Can you work these out from the model? Positions are in its coordinate system, mm. Face numbers are marked on the shaded views. Coordinates: 2 decimals unless noted, no trailing zeros. Order: outer loops, then holes, each group sorted by start corner. A loop starts at its lowest first (then second) coordinate and runs counter-clockwise, first axis right, second up. Notation, with made-up numbers: (-24.75, 39) - (17.25, 39) arc R20 ccw to (17.25, 65) - close; hole circle Ø3 at (7, -13.5). An arc over 180 degrees is marked (long way). Use a Markdown table: item, result. Add a question column.
(1) We'd pull the mould along Z, two halves only. Please class the marked faces 1, 2 and 3: pulls with the +Z half, pulls with the -Z half, needs draft (parallel to the pull), parting line crosses it, or undercut.
(2) If I drill on L1, parallel to Y at x = -12, z = 5; L2, parallel to X at y = 3, z = -3.5; L3, parallel to X at y = 2, z = 14.05, over which ranges is the centre line in solid material (lowest first)? Write a range as [from, to].
(3) For pin 1 Ø1.2 at (y, z) = (1, -12.5) entering from -X; pin 2 Ø1.5 at (y, z) = (1.5, 0) entering from +X; pin 3 Ø1.5 at (x, y) = (-11.5, 1) entering from +Z; pin 4 Ø10 at (x, z) = (-1, -7.5) entering from -Y, each with a flat end and sliding along its axis, tell me the tip position at first contact or that it passes through.
(4) I want a section at B-B (y = 0.75). List the corners of the cut face in (x, z) for me.
```python
from build123d import *

# Parameters (mm, degrees)
EXTRUDE_1_DEPTH          = 4
CUT_EXTRUDE_1_DEPTH      = 31.6757233
CUT_EXTRUDE_1_DEPTH_BACK = 31.6757233
SKETCH_2_R               = 0.5
CUT_EXTRUDE_2_REACH      = 32.237
SKETCH_3_R               = 0.5
FILLET_1_R               = 2
FILLET_2_R               = 1


# Some blends are built 0.0001 mm under size
with BuildPart() as part:
    # Эскиз1 → Бобышка-Вытянуть1 (new body)
    with BuildSketch(Plane(origin=(0, 0, 0), x_dir=(1, 0, 0), z_dir=(0, 1, 0))):
        Polygon((-10, 15), (10, 15), (10, 12), (5, 12), (5, -12), (10, -12), (10, -15), (-10, -15), (-10, -11.5), (-14, -11.5), (-14, 11.5), (-10, 11.5), align=None)
    extrude(amount=EXTRUDE_1_DEPTH)

    # Эскиз2 → Вырез-Вытянуть1 (cut, two sides: drawn at the far end of the back side and taken through both)
    with BuildSketch(Plane.XY.offset(-12).offset(-CUT_EXTRUDE_1_DEPTH_BACK)):
        with Locations((8, 2)):
            Circle(SKETCH_2_R)
    extrude(amount=CUT_EXTRUDE_1_DEPTH + CUT_EXTRUDE_1_DEPTH_BACK, mode=Mode.SUBTRACT)

    # Эскиз3 → Вырез-Вытянуть2 (cut, up to next)
    with BuildSketch(Plane.XY.offset(11.5), mode=Mode.PRIVATE) as cut_extrude_2_sk1:
        with Locations((-12, 2)):
            Circle(SKETCH_3_R)
    cut_extrude_2_tool1 = extrude(cut_extrude_2_sk1.sketch, amount=-CUT_EXTRUDE_2_REACH, mode=Mode.PRIVATE) & part.part
    add(cut_extrude_2_tool1.solids().sort_by_distance((-12, 2, 11.5))[0], mode=Mode.SUBTRACT)

    # Скругление1
    fillet_1_edges = [part.edges().sort_by_distance(p)[0] for p in [
        (10, 0, -13.5),
        (10, 4, -13.5),
        (10, 0, 13.5),
        (10, 4, 13.5),
        (-14, 0, 0),
        (-14, 4, 0),
        (-10, 2, -15),
        (-10, 2, 15),
    ]]
    fillet(fillet_1_edges, radius=FILLET_1_R - 0.0001)  # a hair under: the kernel refuses the full size

    # Скругление2
    # the kernel refuses this fillet: 1 mm, written as the material it takes off along each edge
    with BuildSketch(Plane(origin=(5, 4, -12), x_dir=(-1, 0, 0), z_dir=(0, 0, 1))) as fillet_2_piece_1:
        with BuildLine():
            CenterArc((FILLET_2_R, FILLET_2_R), FILLET_2_R, 180, 90)
            Line((0, FILLET_2_R), (0, 0))
            Line((0, 0), (FILLET_2_R, 0))
        make_face()
    extrude(amount=24, mode=Mode.SUBTRACT)
    with BuildSketch(Plane(origin=(10.5001, 4, -12), x_dir=(0, 0, -1), z_dir=(-1, 0, 0)), Plane(origin=(5, 4, 12), x_dir=(0, 0, 1), z_dir=(1, 0, 0))) as fillet_2_piece_2:
        with BuildLine():
            CenterArc((FILLET_2_R, FILLET_2_R), FILLET_2_R, 180, 90)
            Line((0, FILLET_2_R), (0, 0))
            Line((0, 0), (FILLET_2_R, 0))
        make_face()
    extrude(amount=5.5001, mode=Mode.SUBTRACT)
    with BuildSketch(Plane(origin=(-14.5001, 4, -11.5), x_dir=(0, 0, 1), z_dir=(1, 0, 0)), Plane(origin=(-10, 4, 11.5), x_dir=(0, 0, -1), z_dir=(-1, 0, 0))) as fillet_2_piece_3:
        with BuildLine():
            CenterArc((FILLET_2_R, FILLET_2_R), FILLET_2_R, 180, 90)
            Line((0, FILLET_2_R), (0, 0))
            Line((0, 0), (FILLET_2_R, 0))
        make_face()
    extrude(amount=4.5001, mode=Mode.SUBTRACT)
    with BuildSketch(Plane(origin=(-10, 4, 13.0001), x_dir=(1, 0, 0), z_dir=(0, 0, -1)), Plane(origin=(-10, 4, -11.5), x_dir=(1, 0, 0), z_dir=(0, 0, -1))) as fillet_2_piece_4:
        with BuildLine():
            CenterArc((FILLET_2_R, FILLET_2_R), FILLET_2_R, 180, 90)
            Line((0, FILLET_2_R), (0, 0))
            Line((0, 0), (FILLET_2_R, 0))
        make_face()
    extrude(amount=1.5001, mode=Mode.SUBTRACT)
    with BuildSketch(Plane(origin=(-8.0001, 4, -15), x_dir=(0, -1, 0), z_dir=(1, 0, 0))) as fillet_2_piece_5:
        with BuildLine():
            CenterArc((FILLET_2_R, -FILLET_2_R), FILLET_2_R, 90, 90)
            Line((0, -FILLET_2_R), (0, 0))
            Line((0, 0), (FILLET_2_R, 0))
        make_face()
    extrude(amount=18.5002, mode=Mode.SUBTRACT)
    with BuildSketch(Plane(origin=(10.5001, 4, 15), x_dir=(0, 0, -1), z_dir=(-1, 0, 0))) as fillet_2_piece_6:
        with BuildLine():
            CenterArc((FILLET_2_R, FILLET_2_R), FILLET_2_R, 180, 90)
            Line((0, FILLET_2_R), (0, 0))
            Line((0, 0), (FILLET_2_R, 0))
        make_face()
    extrude(amount=18.5002, mode=Mode.SUBTRACT)
    with BuildSketch(Plane(origin=(-8.0001, 4, 13.0001), x_dir=(0, 0, 1), z_dir=(1, 0, 0))) as fillet_2_piece_7:
        with BuildLine():
            CenterArc((1.9999 - FILLET_2_R, FILLET_2_R), FILLET_2_R, 270, 90)
            Line((1.9999, FILLET_2_R), (1.9999, 0))
            Line((1.9999, 0), (1.9999 - FILLET_2_R, 0))
        make_face()
    revolve(axis=Axis((-8.0001, 4, 13.0001), (0, -1, 0)), revolution_arc=90, mode=Mode.SUBTRACT)
    with BuildSketch(Plane(origin=(-8.0001, 4, -13.0001), x_dir=(0, 0, -1), z_dir=(1, 0, 0))) as fillet_2_piece_8:
        with BuildLine():
            CenterArc((1.9999 - FILLET_2_R, -FILLET_2_R), FILLET_2_R, 0, 90)
            Line((1.9999 - FILLET_2_R, 0), (1.9999, 0))
            Line((1.9999, 0), (1.9999, -FILLET_2_R))
        make_face()
    revolve(axis=Axis((-8.0001, 4, -13.0001), (0, 1, 0)), revolution_arc=90, mode=Mode.SUBTRACT)
    with BuildSketch(Plane(origin=(10.5001, 4, -12), x_dir=(0, 0, -1), z_dir=(-1, 0, 0))) as fillet_2_piece_9a_section:
        with BuildLine():
            CenterArc((FILLET_2_R, FILLET_2_R), FILLET_2_R, 180, 90)
            Line((0, FILLET_2_R), (0, 0))
            Line((0, 0), (FILLET_2_R, 0))
        make_face()
    fillet_2_piece_9a = extrude(amount=8.0001, mode=Mode.PRIVATE)
    fillet_2_piece_9a = split(fillet_2_piece_9a, bisect_by=Plane(origin=(5, 3.773604886, -12.226395114), z_dir=(-1, 0, 0)), keep=Keep.TOP, mode=Mode.PRIVATE)
    with BuildSketch(Plane(origin=(5, 4, -14.5), x_dir=(-1, 0, 0), z_dir=(0, 0, 1))) as fillet_2_piece_9b_section:
        with BuildLine():
            CenterArc((FILLET_2_R, FILLET_2_R), FILLET_2_R, 180, 90)
            Line((0, FILLET_2_R), (0, 0))
            Line((0, 0), (FILLET_2_R, 0))
        make_face()
    fillet_2_piece_9b = extrude(amount=26.5, mode=Mode.PRIVATE)
    fillet_2_piece_9b = split(fillet_2_piece_9b, bisect_by=Plane(origin=(4.773604886, 3.773604886, -12), z_dir=(0, 0, -1)), keep=Keep.TOP, mode=Mode.PRIVATE)
    fillet_2_piece_9 = fillet_2_piece_9a & fillet_2_piece_9b
    add(fillet_2_piece_9, mode=Mode.SUBTRACT)
    with BuildSketch(Plane(origin=(5, 4, -12), x_dir=(-1, 0, 0), z_dir=(0, 0, 1))) as fillet_2_piece_10a_section:
        with BuildLine():
            CenterArc((FILLET_2_R, FILLET_2_R), FILLET_2_R, 180, 90)
            Line((0, FILLET_2_R), (0, 0))
            Line((0, 0), (FILLET_2_R, 0))
        make_face()
    fillet_2_piece_10a = extrude(amount=26.5, mode=Mode.PRIVATE)
    fillet_2_piece_10a = split(fillet_2_piece_10a, bisect_by=Plane(origin=(4.773604886, 3.773604886, 12), z_dir=(0, 0, 1)), keep=Keep.TOP, mode=Mode.PRIVATE)
    with BuildSketch(Plane(origin=(2.5, 4, 12), x_dir=(0, 0, 1), z_dir=(1, 0, 0))) as fillet_2_piece_10b_section:
        with BuildLine():
            CenterArc((FILLET_2_R, FILLET_2_R), FILLET_2_R, 180, 90)
            Line((0, FILLET_2_R), (0, 0))
            Line((0, 0), (FILLET_2_R, 0))
        make_face()
    fillet_2_piece_10b = extrude(amount=8.0001, mode=Mode.PRIVATE)
    fillet_2_piece_10b = split(fillet_2_piece_10b, bisect_by=Plane(origin=(5, 3.773604886, 12.226395114), z_dir=(-1, 0, 0)), keep=Keep.TOP, mode=Mode.PRIVATE)
    fillet_2_piece_10 = fillet_2_piece_10a & fillet_2_piece_10b
    add(fillet_2_piece_10, mode=Mode.SUBTRACT)
    with BuildSketch(Plane(origin=(-10, 4, -9), x_dir=(1, 0, 0), z_dir=(0, 0, -1))) as fillet_2_piece_11a_section:
        with BuildLine():
            CenterArc((FILLET_2_R, FILLET_2_R), FILLET_2_R, 180, 90)
            Line((0, FILLET_2_R), (0, 0))
            Line((0, 0), (FILLET_2_R, 0))
        make_face()
    fillet_2_piece_11a = extrude(amount=4.0001, mode=Mode.PRIVATE)
    fillet_2_piece_11a = split(fillet_2_piece_11a, bisect_by=Plane(origin=(-9.773604886, 3.773604886, -11.5), z_dir=(0, 0, 1)), keep=Keep.TOP, mode=Mode.PRIVATE)
    with BuildSketch(Plane(origin=(-14.5001, 4, -11.5), x_dir=(0, 0, 1), z_dir=(1, 0, 0))) as fillet_2_piece_11b_section:
        with BuildLine():
            CenterArc((FILLET_2_R, FILLET_2_R), FILLET_2_R, 180, 90)
            Line((0, FILLET_2_R), (0, 0))
            Line((0, 0), (FILLET_2_R, 0))
        make_face()
    fillet_2_piece_11b = extrude(amount=7.0001, mode=Mode.PRIVATE)
    fillet_2_piece_11b = split(fillet_2_piece_11b, bisect_by=Plane(origin=(-10, 3.773604886, -11.273604886), z_dir=(1, 0, 0)), keep=Keep.TOP, mode=Mode.PRIVATE)
    fillet_2_piece_11 = fillet_2_piece_11a & fillet_2_piece_11b
    add(fillet_2_piece_11, mode=Mode.SUBTRACT)
    with BuildSketch(Plane(origin=(-7.5, 4, 11.5), x_dir=(0, 0, -1), z_dir=(-1, 0, 0))) as fillet_2_piece_12a_section:
        with BuildLine():
            CenterArc((FILLET_2_R, FILLET_2_R), FILLET_2_R, 180, 90)
            Line((0, FILLET_2_R), (0, 0))
            Line((0, 0), (FILLET_2_R, 0))
        make_face()
    fillet_2_piece_12a = extrude(amount=7.0001, mode=Mode.PRIVATE)
    fillet_2_piece_12a = split(fillet_2_piece_12a, bisect_by=Plane(origin=(-10, 3.773604886, 11.273604886), z_dir=(1, 0, 0)), keep=Keep.TOP, mode=Mode.PRIVATE)
    with BuildSketch(Plane(origin=(-10, 4, 13.0001), x_dir=(1, 0, 0), z_dir=(0, 0, -1))) as fillet_2_piece_12b_section:
        with BuildLine():
            CenterArc((FILLET_2_R, FILLET_2_R), FILLET_2_R, 180, 90)
            Line((0, FILLET_2_R), (0, 0))
            Line((0, 0), (FILLET_2_R, 0))
        make_face()
    fillet_2_piece_12b = extrude(amount=4.0001, mode=Mode.PRIVATE)
    fillet_2_piece_12b = split(fillet_2_piece_12b, bisect_by=Plane(origin=(-9.773604886, 3.773604886, 11.5), z_dir=(0, 0, -1)), keep=Keep.TOP, mode=Mode.PRIVATE)
    fillet_2_piece_12 = fillet_2_piece_12a & fillet_2_piece_12b
    add(fillet_2_piece_12, mode=Mode.SUBTRACT)


solid = part.part
```
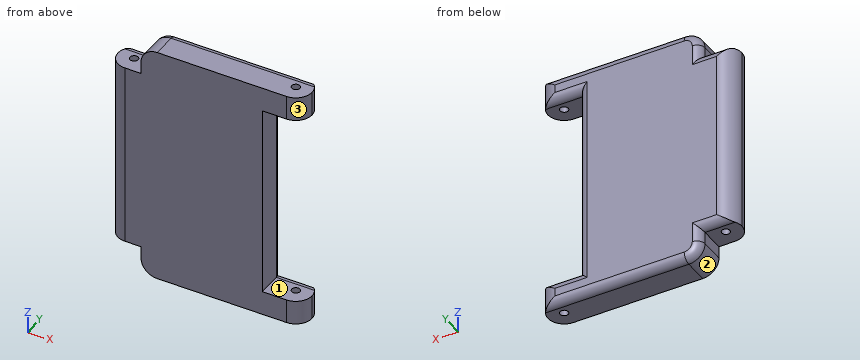
Answers follow:
| question | item | result |
|---|---|---|
| 1 | face 1 | undercut |
| 1 | face 2 | pulls with the -Z half |
| 1 | face 3 | needs draft |
| 2 | L1 | y = [0, 1.5], [2.5, 4] |
| 2 | L2 | x = [-13.73, 5] |
| 2 | L3 | x = [-9.7, 7.5], [8.5, 10] |
| 3 | pin 1 | stops at x = -10 |
| 3 | pin 2 | stops at x = 5 |
| 3 | pin 3 | stops at z = 11.5 |
| 3 | pin 4 | stops at y = 0 |
| 4 | outline | (-13.56, -11.5) - (-10, -11.5) - (-10, -13) arc R2 ccw to (-8, -15) - (9.56, -15) - (9.56, -12) - (5, -12) - (5, 12) - (9.56, 12) - (9.56, 15) - (-8, 15) arc R2 ccw to (-10, 13) - (-10, 11.5) - (-13.56, 11.5) - close |
